```python
from build123d import *

# Parameters (mm, degrees)
SKETCH1_W           = 45
SKETCH1_H           = 60
BOSS_EXTRUDE1_DEPTH = 15
SKETCH2_R           = 4
SKETCH2_W           = 10
SKETCH2_H           = 25
CUT_EXTRUDE1_DEPTH  = 46
SKETCH3_W           = 17
SKETCH3_H           = 12
BOSS_EXTRUDE2_DEPTH = 45
SKETCH4_W           = 25
SKETCH4_H           = 17
BOSS_EXTRUDE3_DEPTH = 18
SKETCH5_W           = 2
SKETCH5_H           = 30
CUT_EXTRUDE2_DEPTH  = 5
SKETCH6_R           = 4.5
CUT_EXTRUDE3_DEPTH  = 61
SKETCH7_R           = 7.5
SKETCH7_R_2         = 5
SKETCH7_R_3         = 1.25
CUT_EXTRUDE4_DEPTH  = 27
SKETCH8_R           = 15
SKETCH8_R_2         = 1.5
CUT_EXTRUDE5_DEPTH  = 22
FILLET1_R           = 6
SKETCH9_R           = 1.5
CUT_EXTRUDE6_DEPTH  = 15


with BuildPart() as part:
    # Sketch1 → Boss-Extrude1 (new body)
    with BuildSketch(Plane.XY):
        Rectangle(SKETCH1_W, SKETCH1_H)
    extrude(amount=BOSS_EXTRUDE1_DEPTH)

    # Sketch2 → Cut-Extrude1 (cut, through all)
    with BuildSketch(Plane(origin=(22.5, 0, 0), x_dir=(0, 0, -1), z_dir=(1, 0, 0))):
        with Locations((-7.5, 22.5)):
            Circle(SKETCH2_R)
        with Locations((-7.5, -22.5)):
            Circle(SKETCH2_R)
        with Locations((-7.5, 0)):
            Rectangle(SKETCH2_W, SKETCH2_H)
    extrude(amount=-CUT_EXTRUDE1_DEPTH, mode=Mode.SUBTRACT)

    # Sketch3 → Boss-Extrude2 (add)
    with BuildSketch(Plane.ZY.offset(22.5)):
        with Locations((23.5, -24)):
            Rectangle(SKETCH3_W, SKETCH3_H)
    extrude(amount=-BOSS_EXTRUDE2_DEPTH)

    # Sketch4 → Boss-Extrude3 (add)
    with BuildSketch(Plane(origin=(0, -18, 0), x_dir=(1, 0, 0), z_dir=(0, 1, 0))):
        with Locations((-10, -23.5)):
            Rectangle(SKETCH4_W, SKETCH4_H)
    extrude(amount=BOSS_EXTRUDE3_DEPTH)

    # Sketch5 → Cut-Extrude2 (cut)
    with BuildSketch(Plane.XY.offset(32)):
        with Locations((-10, -15)):
            Rectangle(SKETCH5_W, SKETCH5_H)
    extrude(amount=-CUT_EXTRUDE2_DEPTH, mode=Mode.SUBTRACT)

    # Sketch6 → Cut-Extrude3 (cut, through all)
    with BuildSketch(Plane.XZ.offset(30)):
        with Locations((-10, 23)):
            Circle(SKETCH6_R)
    extrude(amount=-CUT_EXTRUDE3_DEPTH, mode=Mode.SUBTRACT)

    # Sketch7 → Cut-Extrude4 (cut)
    with BuildSketch(Plane.XZ.offset(30)):
        with Locations((-10, 23)):
            Circle(SKETCH7_R)
        with Locations((11.1, 23)):
            Circle(SKETCH7_R_2)
        with Locations((18.6, 23)):
            Circle(SKETCH7_R_3)
        with Locations((11.1, 30.5)):
            Circle(SKETCH7_R_3)
        with Locations((11.1, 15.5)):
            Circle(SKETCH7_R_3)
        with Locations((3.6, 23)):
            Circle(SKETCH7_R_3)
    extrude(amount=-CUT_EXTRUDE4_DEPTH, mode=Mode.SUBTRACT)

    # Sketch8 → Cut-Extrude5 (cut)
    with BuildSketch(Plane(origin=(0, 0, 0), x_dir=(-1, 0, 0), z_dir=(0, 0, -1))):
        with Locations((2.5, 0)):
            Circle(SKETCH8_R)
        with Locations((18.25, 15.75)):
            Circle(SKETCH8_R_2)
        with Locations((-13.25, 15.75)):
            Circle(SKETCH8_R_2)
        with Locations((-13.25, -15.75)):
            Circle(SKETCH8_R_2)
        with Locations((18.25, -15.75)):
            Circle(SKETCH8_R_2)
    extrude(amount=-CUT_EXTRUDE5_DEPTH, mode=Mode.SUBTRACT)

    # Fillet1
    fillet1_edges = [part.edges().sort_by_distance(p)[0] for p in [
        (-22.5, -15, 32),
        (22.5, -24, 32),
        (2.5, -9, 32),
    ]]
    fillet(fillet1_edges, radius=FILLET1_R)

    # Sketch9 → Cut-Extrude6 (cut)
    with BuildSketch(Plane(origin=(0, 0, 0), x_dir=(-1, 0, 0), z_dir=(0, 0, -1))):
        with Locations((-18, 0)):
            Circle(SKETCH9_R)
    extrude(amount=-CUT_EXTRUDE6_DEPTH, mode=Mode.SUBTRACT)


solid = part.part
```
Verification items for the finished model (mm, model axes). A direction names the side the tool comes from. Give positions to 0.01 mm unless a question says otherwise; leave off trailing zeros. Order: outer loops, then holes, each group sorted by start corner. A loop starts at its lowest first (then second) coordinate and runs counter-clockwise, first axis right, second up. Notation, with made-up numbers: (5, 9) - (18, 9) arc R24 ccw to (18, 27) - close; hole circle Ø11 at (-3.75, 26.25). An arc over 180 degrees is marked (long way). Answer as CSV lines item,"result". Start each with the question number.
Item 1: Gauge pin test, flat ends, axial feed: pin 1 (1.5 mm diameter, centred on x = 5.5, z = 16, fed in from +Y); pin 2 (0.7 mm diameter, centred on x = -18.5, y = -15.5, fed in from -Z); pin 3 (13.5 mm diameter, centred on x = 4, z = 22.5, fed in from +Y). Record the tip position at first contact, or that the pin passes through.
Item 2: Section check C-C, the plane y = 2.5. Record the boundary of the cut face in (x, z), plus the area to 3 significant figures.
Item 3: Material ranges on L1, parallel to Y at x = 10, z = 7.5; L2, parallel to X at y = -14.5, z = 23; L3, parallel to Z at x = 17, y = 1.5, recorded low to high.
Item 4: Section check D-D, the plane x = 13.25. Record the boundary of the cut face in (y, z), plus the area to 3 significant figures.
Item 5: Section check B-B, the plane x = -10. Record the boundary of the cut face in (y, z).
Item 6: Access from +Z, -Z, +X, -X, +Y, -Y to the whole of each face (thin tool, end or side, straight path). Record for faces 1 (the face through (-19, 0, 12.5)), 2 (the face through (-11, -12, 31)), 3 (the face through (10.83, -22.69, 14.28)), 4 (the face through (-22.5, -7, 13)), 5 (the face through (15, -18, 27)).
Item 7: Section check A-A, the plane x = 18.6. Record the boundary of the cut face in (y, z).
Item 8: Mould release check, pull along Y, two halves, no side actions. Record for faces 6 (the face through (14.75, 15.82, 7.4)), 7 (the face through (7, -15, 15)), 8 (the face through (-3, 0, 27)): released by +Y, released by -Y, zero draft, split by the parting line, or undercut.
Filled in:
1,pin 1,"y = -18"
1,pin 2,"z = 22"
1,pin 3,"y = 0"
2,outline,"(-22.5, 0) - (-17.29, 0) - (-17.29, 2.5) - (-22.5, 2.5) - close; (-22.5, 12.5) - (-17.29, 12.5) - (-17.29, 15) - (-22.5, 15) - close; (12.29, 0) - (22.5, 0) - (22.5, 2.5) - (12.29, 2.5) - close; (12.29, 12.5) - (22.5, 12.5) - (22.5, 15) - (12.29, 15) - close"
2,area,"77.1 mm^2"
3,L1,"-30 to -26.5, -18.5 to -12.5, 12.5 to 18.5, 26.5 to 30"
3,L2,"-22.5 to -17.5, -2.5 to 2.35"
3,L3,"0 to 2.5, 12.5 to 15"
4,outline,"(-30, 0) - (-17.25, 0) - (-17.25, 15) - (-18, 15) - (-18, 18.49) - (-30, 18.49) - close; (-30, 27.51) - (-18, 27.51) - (-18, 32) - (-30, 32) - close; (-14.25, 0) - (14.25, 0) - (14.25, 15) - (-14.25, 15) - close; (17.25, 0) - (30, 0) - (30, 15) - (17.25, 15) - close; hole circle Ø8 at (-22.5, 7.5); hole (-12.5, 2.5) - (12.5, 2.5) - (12.5, 12.5) - (-12.5, 12.5) - close; hole circle Ø8 at (22.5, 7.5)"
4,area,"555 mm^2"
5,outline,"(-30, 0) - (-12.99, 0) - (-12.99, 15.5) - (-30, 15.5) - close; (12.99, 0) - (30, 0) - (30, 15) - (12.99, 15) - close; hole circle Ø8 at (-22.5, 7.5); hole circle Ø8 at (22.5, 7.5)"
6,face 1,"+X, -X"
6,face 2,"+Z, +Y, -Y"
6,face 3,"-Y"
6,face 4,"+Z, -Z, -X, +Y, -Y"
6,face 5,"+Z, +X, +Y"
7,outline,"(-30, 0) - (-1.37, 0) - (-1.37, 2.5) - (-12.5, 2.5) - (-12.5, 12.5) - (-1.37, 12.5) - (-1.37, 15) - (-18, 15) - (-18, 21.75) - (-30, 21.75) - close; (-30, 24.25) - (-18, 24.25) - (-18, 31.62) - (-30, 31.62) - close; (1.37, 0) - (30, 0) - (30, 15) - (1.37, 15) - (1.37, 12.5) - (12.5, 12.5) - (12.5, 2.5) - (1.37, 2.5) - close; hole circle Ø8 at (-22.5, 7.5); hole circle Ø8 at (22.5, 7.5)"
8,face 6,"undercut"
8,face 7,"zero draft"
8,face 8,"released by +Y"
